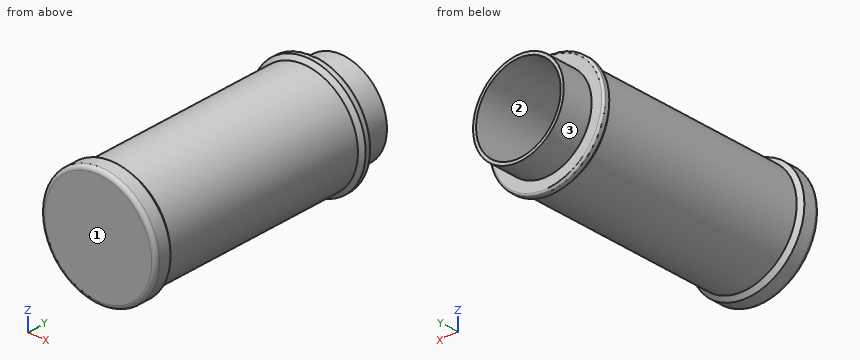
Autodesk Inventor part; units mm, degrees
ref_plane "Work Plane2" through (0, 0, 0) normal (0, 0, 1) x (1, 0, 0)
ref_plane "YZ Plane" through (0, 0, 0) normal (1, 0, 0) x (0, 1, 0)
ref_plane "XZ Plane" through (0, 0, 0) normal (0, 1, 0) x (-1, 0, 0)
sketch "Sketch1" plane through (0, 0, 0) normal (0, 1, 0) x (-1, 0, 0)
  circle A0 centre (0, 0) radius 28.5
  dimension "d0" = 57
extrude "Extrusion1" add sketch "Sketch1" along normal blind 131
sketch "Sketch2" plane through (0, 131, 0) normal (0, 1, 0) x (1, 0, 0)
  circle A0 centre (0, 0) radius 25
  circle A1 centre (0, 0) radius 22.5
  circle A2 centre (0, 0) radius 28.5
  dimension "d3" = 50
  dimension "d4" = 45
  dimension "d8" = 57
extrude "Extrusion2" cut sketch "Sketch2" against normal blind 15 contours A0 | A2
ref_plane "Work Plane2" through (0, 0, 0) normal (0, 0, 1) x (1, 0, 0)
sketch "Sketch4" plane through (0, 0, 0) normal (0, 0, 1) x (1, 0, 0)
  line L0 (28.5, 0) -> (28.5, 116)
  line L1 (-28.5, 116) -> (28.5, 116)
  line L2 (28.5, 116) -> (28.5, 111)
  line L3 (28.5, 111) -> (26.5, 111)
  line L4 (28.5, 0) -> (-28.5, 0)
  line L5 (28.5, 0) -> (28.5, 10)
  line L6 (28.5, 10) -> (26.5, 10)
  line L7 (26.5, 10) -> (26.5, 111)
  line L8 (28.5, 111) -> (28.5, 10)
  line L9 (0, -23.2) -> (0, 139.2)
  point P0 (0, 0)
  dimension "d10" = 5
  dimension "d11" = 2
  dimension "d12" = 10
  dimension "d13" = 2
revolve "Revolution1" cut sketch "Sketch4" angle 360 about axis through (0, -10, 0) along (0, 1, 0) contours L6 L7 L3 L0
chamfer "Chamfer1" distance 2 angle 45 1 edges at (28.5, 10, 0)
chamfer "Chamfer2" distance 2 angle 45 1 edges at (28.5, 111, 0)
fillet "Fillet1" radius 2 1 edges at (28.5, 0, 0)
fillet "Fillet2" radius 1 1 edges at (28.5, 116, 0)
sketch "Sketch5" plane through (0, 0, 0) normal (0, 0, 1) x (1, 0, 0)
  point P0 (0, 0)
sketch "Sketch6" plane through (0, 131, 0) normal (0, 1, 0) x (1, 0, 0)
  circle A0 centre (0, 0) radius 21
  dimension "d27" = 42
extrude "Extrusion3" cut sketch "Sketch6" against normal blind 125
properties part number "FiestaSpiceContainer"
Could you check a few things on this model? Use its own coordinates, in mm. Face numbers are marked on the shaded views. Coordinates: 2 decimals unless noted, no trailing zeros. Order: outer loops, then holes, each group sorted by start corner. A loop starts at its lowest first (then second) coordinate and runs counter-clockwise, first axis right, second up.
Q1. Thinking about a two-plate mould opening in X: for the marked faces 1, 2 and 3, which applies, released by +X, released by -X, zero draft, split by the parting line, or undercut?
Q2. Will these pins go through, and if not, where does the flat tip stop? pin 1 (6 mm diameter, centred on x = 21.5, y = 25.5, fed in from +Z); pin 2 (10 mm diameter, centred on y = 89.5, z = -21.5, fed in from -X); pin 3 (8 mm diameter, centred on y = 43.5, z = -2, fed in from +X).
Q3. Suppose I cut it at C-C on y = 44. Please give me the cut outline in (x, z), and give its area (3 significant figures).
Q4. Please list where these lines run through material, in increasing order: L1, parallel to Z at x = -1, y = 49.5; L2, parallel to X at y = 71.5, z = 0; L3, parallel to Y at x = 10, z = 9.
Answer:
1. face 1: zero draft
1. face 2: undercut
1. face 3: split by the parting line
2. pin 1: stops at z = 18.97
2. pin 2: stops at x = -20.74
2. pin 3: stops at x = 26.5
3. outline: circle Ø53 at (0, 0); hole circle Ø42 at (0, 0)
3. area: 821 mm2
4. L1: z = -26.48 to -20.98, 20.98 to 26.48
4. L2: x = -26.5 to -21, 21 to 26.5
4. L3: y = 0 to 6
